Verification items for the finished model (mm, model axes). A direction names the side the tool comes from. Coordinates: 2 decimals unless noted, no trailing zeros. Write each loop counter-clockwise with the first axis right and the second up, starting at its lowest first coordinate (ties: lowest second). Pieces come first, ordered by that corner, then holes. Notation, with made-up numbers: (-30, 25) - (27, 25) arc R17 ccw to (27, 51) - close; hole circle Ø1 at (32, -5). An arc over 180 degrees is marked (long way). Use one line per item in the form item = value. Start each with the question number.
(1) Material ranges on line 1 (Z direction, x = 8.75, y = -6.5); line 2 (X direction, y = 14.5, z = 1); line 3 (Y direction, x = -4.75, z = 6.75), recorded low to high. Write a range as [from, to].
(2) Sectioned sample at B-B (x = 0). Record the cut outline in (y, z), and give its area (3 significant figures).
(3) Mould release check, pull along X, two halves, no side actions. Record for faces 1 (the flat face through (-9.779, 0, 5)), 2 (the cylindrical face through (-7.593, 21.838, 1.615)), 3 (the flat face through (0, -22.892, 2)), 4 (the flat face through (10.541, 0, 2)): released by +X, released by -X, zero draft, split by the parting line, or undercut.
(4) Gauge pin test, flat ends, axial feed: pin 1 Ø8 at (x, z) = (-14, 6) entering from -Y; pin 2 Ø1.5 at (x, y) = (-10, 17.5) entering from +Z; pin 3 Ø0.8 at (x, z) = (-11, 4.5) entering from +Y; pin 4 Ø5 at (x, y) = (-11.5, 15.5) entering from -Z. Record the tip position at first contact, or that the pin passes through.
(5) Tool access check on faces 5 (the flat face through (-11, 0, 3.277)), 6 (the flat face through (-11, 3.842, 5)), 7 (the cylindrical face through (7.63, -7.96, 9.54)), 8 (the flat face through (-11, -3.778, 5)), 9 (the flat face through (-11, 0, 5.817)). Record the directions out of +Z, -Z, +X, -X, +Y, -Y that give a thin tool (end or side, any length) a straight path to the whole face; none if there is none.
(6) Sectioned sample at A-A (x = -16.25). Record the cut outline in (y, z), and give its area (3 significant figures).
(7) Sectioned sample at D-D (y = 8). Record the cut outline in (x, z).
(8) Sectioned sample at C-C (z = 1.75). Count the separate pieces of the cut face and the enclosed holes in it, and give its area (3 significant figures).
from build123d import *

# Parameters (mm, degrees)
SKETCH1_W           = 45.7835
SKETCH1_H           = 21.082
SKETCH1_R           = 1.5875
BOSS_EXTRUDE1_DEPTH = 3.2766
SKETCH2_R           = 8.001
BOSS_EXTRUDE2_DEPTH = 12.7
SKETCH3_W           = 2.54
SKETCH3_H           = 7.62
BOSS_EXTRUDE3_DEPTH = 2.54
SKETCH4_W           = 0.635
SKETCH4_H           = 0.635
BOSS_EXTRUDE4_DEPTH = 6.35


with BuildPart() as part:
    # Sketch1 → Boss-Extrude1 (new body)
    with BuildSketch(Plane(origin=(0, 0, 0), x_dir=(0, 1, 0), z_dir=(0, 0, 1))):
        Rectangle(SKETCH1_W, SKETCH1_H)
        with Locations(Location((-20.28825, -7.9375, 0), (0, 0, 90))):
            Circle(SKETCH1_R, mode=Mode.SUBTRACT)
        with Locations(Location((20.28825, 7.9375, 0), (0, 0, 90))):
            Circle(SKETCH1_R, mode=Mode.SUBTRACT)
    extrude(amount=BOSS_EXTRUDE1_DEPTH)

    # Sketch2 → Boss-Extrude2 (add)
    with BuildSketch(Plane.XY.offset(3.2766)):
        with Locations((0, 10.362469871)):
            Circle(SKETCH2_R)
        with Locations((0, -10.362469871)):
            Circle(SKETCH2_R)
    extrude(amount=BOSS_EXTRUDE2_DEPTH)

    # Sketch3 → Boss-Extrude3 (add)
    with BuildSketch(Plane.XY.offset(3.2766)):
        with Locations((-11.049, 0.03175)):
            Rectangle(SKETCH3_W, SKETCH3_H)
    extrude(amount=BOSS_EXTRUDE3_DEPTH)

    # Sketch4 → Boss-Extrude4 (add)
    with BuildSketch(Plane(origin=(-12.319, 0, 0), x_dir=(0, -1, 0), z_dir=(-1, 0, 0))):
        with Locations((2.50825, 4.5466)):
            Rectangle(SKETCH4_W, SKETCH4_H)
        with Locations((-0.03175, 4.5466)):
            Rectangle(SKETCH4_W, SKETCH4_H)
        with Locations((-2.57175, 4.5466)):
            Rectangle(SKETCH4_W, SKETCH4_H)
    extrude(amount=BOSS_EXTRUDE4_DEPTH)


solid = part.part
Answers below:
q1.line_1 = [0, 3.28]
q1.line_2 = [-10.54, 10.54]
q1.line_3 = [-16.8, -3.92], [3.92, 16.8]
q2.outline = (-22.89, 0) - (22.89, 0) - (22.89, 3.28) - (18.36, 3.28) - (18.36, 15.98) - (2.36, 15.98) - (2.36, 3.28) - (-2.36, 3.28) - (-2.36, 15.98) - (-18.36, 15.98) - (-18.36, 3.28) - (-22.89, 3.28) - close
q2.area = 556 mm2
q3.face_1 = undercut
q3.face_2 = undercut
q3.face_3 = zero draft
q3.face_4 = released by +X
q4.pin_1 = -3.78
q4.pin_2 = 3.28
q4.pin_3 = 3.84
q4.pin_4 = 0
q5.face_5 = -Z, -X, +Y, -Y
q5.face_6 = +Z, -X, +Y
q5.face_7 = +Z
q5.face_8 = +Z, -X, -Y
q5.face_9 = +Z, -X, +Y, -Y
q6.outline = (-2.83, 4.23) - (-2.19, 4.23) - (-2.19, 4.86) - (-2.83, 4.86) - close; (-0.29, 4.23) - (0.35, 4.23) - (0.35, 4.86) - (-0.29, 4.86) - close; (2.25, 4.23) - (2.89, 4.23) - (2.89, 4.86) - (2.25, 4.86) - close
q6.area = 1.21 mm2
q7.outline = (-10.54, 0) - (10.54, 0) - (10.54, 3.28) - (7.64, 3.28) - (7.64, 15.98) - (-7.64, 15.98) - (-7.64, 3.28) - (-10.54, 3.28) - close
q8.separate_pieces = 1
q8.enclosed_holes = 2
q8.area = 949 mm2
